Work out the finished part from the listing and answer in its coordinate system (mm). A direction names the side the tool comes from. Round coordinates to 2 decimals unless told otherwise and drop trailing zeros. Write each loop counter-clockwise with the first axis right and the second up, starting at its lowest first coordinate (ties: lowest second). Pieces come first, ordered by that corner, then holes. Notation, with made-up numbers: (-35, 26) - (22, 26) arc R20 cw to (22, 33) - close; hole circle Ø2 at (-15, 75). An arc over 180 degrees is marked (long way). Answer as a JSON object with one key per item and string values.
```python
from build123d import *

# Parameters (mm, degrees)
F1_DEPTH = 50.8
F2_W     = 153.3701941371
F2_H     = 109.4799749553
F3_DEPTH = 25.4
F4_T     = -2.54


# Not quite as in the source:
# - a shell that OpenCascade refuses in one call is made with other operations: the cavity is built on its own and cut out


with BuildPart() as f1:
    # F0 (on Top) → F1 (new body)
    with BuildSketch(Plane.XY):
        Polygon((32.5404184413, -50.9185224387), (60.4496595907, 2.769324145), (27.9092411494, 53.7833592726), (-32.5404184413, 51.1095478164), (-60.4496595907, -2.5782987673), (-27.9092411494, -53.5923338949), align=None)
    extrude(amount=F1_DEPTH)

    # F2 (on Front) → F3 (join)
    with BuildSketch(Plane.XZ):
        with Locations((0.9111128747, 20.3165654093)):
            Rectangle(F2_W, F2_H)
    extrude(amount=F3_DEPTH)

    # F4: a shell. OpenCascade refuses it in one call, so the cavity is built on its own and cut out:
    # the body offset inwards by the wall thickness, plus a prism from it out through each open face.
    f4_core = offset(f1.part, amount=F4_T, kind=Kind.INTERSECTION, mode=Mode.PRIVATE)
    f4_exits = [f4_core.faces().sort_by_distance(p)[0] for p in [
        (0.261081, -35.353201, 48.26),
    ]]
    add(f4_core, mode=Mode.SUBTRACT)
    extrude(f4_exits, amount=-F4_T, mode=Mode.SUBTRACT)


solid = f1.part
```
Item 1: Each of these flat-tipped pins is pushed along its axis until it touches: P1, Ø16, axis at x = -10, y = 30.5, coming from the -Z side; P2, Ø10, axis at x = -9.5, y = 9.5, coming from the +Z side; P3, Ø6, axis at x = -6, z = 53, coming from the -Y side. Where does it stop, or does it pass through?
Results found:
{"P1": "z = 0", "P2": "z = 50.8", "P3": "y = -52.71"}
Item 2: A cutting plane is placed at C-C (y = -45). Write down the section's boundary in (x, z), and give its area (3 significant figures).
Results found:
{"outline": "(-33.39, 0) - (35.62, 0) - (35.62, 50.8) - (32.75, 50.8) - (32.75, 2.54) - (-30.38, 2.54) - (-30.38, 50.8) - (-33.39, 50.8) - close", "area": "459 mm²"}
Item 3: Consider line 1 along Z through (x, y) = (41, 15.5); line 2 along Y through (x, z) = (-59, 60); line 3 along X through (y, z) = (-7.5, 38). Determine where each line is inside the solid, lowest interval first.
Results found:
{"line 1": "0 to 2.54, 48.26 to 50.8", "line 2": "-25.4 to -22.86, -2.54 to 0", "line 3": "-75.77 to -73.23, 75.06 to 77.6"}
Item 4: Determine the mould class of faces 4 (the flat face through (0, 21, 50.8)), 5 (the flat face through (0, -25.4, -3)), 6 (the flat face through (-1, 19, 48.26)) for opening direction Z: pulls with the +Z half, pulls with the -Z half, needs draft (parallel to the pull), parting line crosses it, or undercut.
Results found:
{"face 4": "pulls with the +Z half", "face 5": "needs draft", "face 6": "undercut"}
Item 5: For faces 1 (the flat face through (0, -50, 50.8)), 2 (the flat face through (-1, -39, 0)), 3 (the flat face through (0, 21, 0)), determine the directions among +Z, -Z, +X, -X, +Y, -Y from which every point of the face is accessible in a straight line to the end or side of a thin tool.
Results found:
{"face 1": "+Z, +X, -X, -Y", "face 2": "-Z, +X, -X, -Y", "face 3": "-Z, +X, -X, +Y"}
Item 6: A cutting plane is placed at A-A (z = -25.5). Write down the section's boundary in (x, y).
Results found:
{"outline": "(-75.77, -25.4) - (77.6, -25.4) - (77.6, 0) - (-75.77, 0) - close; hole (-73.23, -22.86) - (75.06, -22.86) - (75.06, -2.54) - (-73.23, -2.54) - close"}
Item 7: A cutting plane is placed at D-D (x = 2). Write down the section's boundary in (y, z).
Results found:
{"outline": "(-52.27, 0) - (-25.4, 0) - (-25.4, -34.42) - (0, -34.42) - (0, 0) - (52.64, 0) - (52.64, 50.8) - (0, 50.8) - (0, 75.06) - (-25.4, 75.06) - (-25.4, 50.8) - (-22.86, 50.8) - (-22.86, 72.52) - (-2.54, 72.52) - (-2.54, 48.26) - (50.09, 48.26) - (50.09, 2.54) - (-2.54, 2.54) - (-2.54, -31.88) - (-22.86, -31.88) - (-22.86, 2.54) - (-49.73, 2.54) - (-49.73, 50.8) - (-52.27, 50.8) - close"}
Item 8: A cutting plane is placed at B-B (y = -13). Write down the section's boundary in (x, z), and give its area (3 significant figures).
Results found:
{"outline": "(-75.77, -34.42) - (77.6, -34.42) - (77.6, 75.06) - (-75.77, 75.06) - close; hole (-73.23, -31.88) - (75.06, -31.88) - (75.06, 72.52) - (-73.23, 72.52) - close", "area": "1,310 mm²"}
